Geometry check sheet. Reference: the model listing, model coordinates, mm. Face numbers are marked on the shaded views. A direction names the side the tool comes from. Coordinates: 2 decimals unless noted, no trailing zeros. Loops run counter-clockwise (first coordinate to the right, second up) from the corner with the lowest first, then second, coordinate; pieces in that order, holes last.
from build123d import *

# Parameters (mm, degrees)
BOSS_EXTRUDE1_DEPTH = 10
FILLET1_R           = 3
SKETCH2_R           = 1.4
CUT_EXTRUDE1_DEPTH  = 58.606674312


with BuildPart() as part:
    # Sketch1 → Boss-Extrude1 (new body)
    with BuildSketch(Plane(origin=(0, 0, 0), x_dir=(1, 0, 0), z_dir=(0, 1, 0))):
        with BuildLine():
            Line((7.5, -36.300826437), (7.5, -46.300826437))
            ThreePointArc((7.5, -46.300826437), (0, -53.800826437), (-7.5, -46.300826437))
            Line((-7.5, -46.300826437), (-7.5, -36.300826437))
            ThreePointArc((-7.5, -36.300826437), (-9.468913253, -22.407853181), (-15.220588235, -9.609042292))
            ThreePointArc((-15.220588235, -9.609042292), (0, 18), (15.220588235, -9.609042292))
            ThreePointArc((15.220588235, -9.609042292), (9.468913253, -22.407853181), (7.5, -36.300826437))
        make_face()
    extrude(amount=BOSS_EXTRUDE1_DEPTH)

    # Fillet1
    fillet1_edges = [part.edges().sort_by_distance(p)[0] for p in [
        (-9.468913253, 10, 22.407853181),
        (-7.5, 10, 41.300826437),
        (0, 10, 53.800826437),
        (7.5, 10, 41.300826437),
        (9.468913253, 10, 22.407853181),
        (7.5, 0, 41.300826437),
        (0, 0, 53.800826437),
        (-7.5, 0, 41.300826437),
        (-9.468913253, 0, 22.407853181),
        (0, 0, -18),
        (9.468913253, 0, 22.407853181),
        (0, 10, -18),
    ]]
    fillet(fillet1_edges, radius=FILLET1_R)

    # Sketch2 → Cut-Extrude1 (cut, through all)
    with BuildSketch(Plane(origin=(0, 10, 0), x_dir=(1, 0, 0), z_dir=(0, 1, 0))):
        with Locations(Location((0, 13.5, 0), (0, 0, 270))):
            Circle(SKETCH2_R)
        with Locations(Location((-11.691342951, -6.75, 0), (0, 0, 270))):
            Circle(SKETCH2_R)
        with Locations(Location((11.691342951, -6.75, 0), (0, 0, 270))):
            Circle(SKETCH2_R)
    extrude(amount=-CUT_EXTRUDE1_DEPTH, mode=Mode.SUBTRACT)


solid = part.part
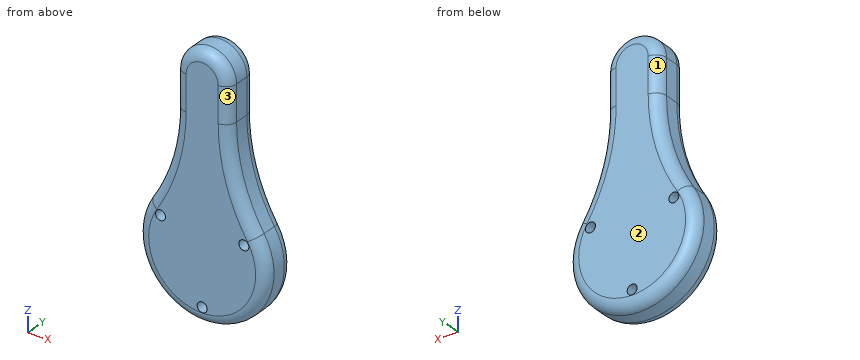
(1) Scan lines: L1, parallel to X at y = 6, z = 6.75; L2, parallel to X at y = 3.75, z = 44; L3, parallel to Z at x = -11, y = 1. Record each from-to range of solid material in increasing order.
Findings:
L1: x = -16.69 to -13.09, -10.29 to 10.29, 13.09 to 16.69
L2: x = -7.5 to 7.5
L3: z = -13.27 to 5.53, 7.97 to 15.94
(2) Gauge pin test, flat ends, axial feed: pin 1 Ø1.2 at (y, z) = (5, 42) entering from +X; pin 2 Ø6 at (x, y) = (-14.5, 7.5) entering from +Z; pin 3 Ø12 at (x, z) = (12, 35.5) entering from -Y. Record the tip position at first contact, or that the pin passes through.
Findings:
pin 1: stops at x = 7.5
pin 2: stops at z = 16.65
pin 3: stops at y = 0.4
(3) Sectioned sample at D-D on z = 6.5. State how many separate pieces and enclosed holes the cut face has, and give its area (3 significant figures).
Findings:
separate pieces: 3
enclosed holes: 0
area: 272 mm2
(4) Access from +Z, -Z, +X, -X, +Y, -Y to the whole of each face (thin tool, end or side, straight path). Record for the marked faces 1, 2 and 3.
Findings:
face 1: +Z, -X, +Y
face 2: +Z, -Z, +X, -X, +Y
face 3: +Z, +X, -Y
(5) Sectioned sample at A-A on x = 0. Record the cut outline in (y, z), and give its area (3 significant figures).
Findings:
outline: (0, -15) arc R3 ccw to (3, -18) - (7, -18) arc R3 ccw to (10, -15) - (10, -14.9) - (0, -14.9) - close; (0, -12.1) - (10, -12.1) - (10, 50.8) arc R3 ccw to (7, 53.8) - (3, 53.8) arc R3 ccw to (0, 50.8) - close
area: 682 mm2
(6) Sectioned sample at C-C on y = 4. Record the cut outline in (x, z), and give its area (3 significant figures).
Findings:
outline: (-15.22, 9.61) arc R18 ccw (long way) to (15.22, 9.61) arc R50 cw to (7.5, 36.3) - (7.5, 46.3) arc R7.5 ccw to (-7.5, 46.3) - (-7.5, 36.3) arc R50 cw to start; hole circle Ø2.8 at (-11.69, 6.75); hole circle Ø2.8 at (0, -13.5); hole circle Ø2.8 at (11.69, 6.75)
area: 1,590 mm2
(7) Sectioned sample at B-B on z = 40. Record the cut outline in (x, y), and give its area (3 significant figures).
Findings:
outline: (-7.5, 3) arc R3 ccw to (-4.5, 0) - (4.5, 0) arc R3 ccw to (7.5, 3) - (7.5, 7) arc R3 ccw to (4.5, 10) - (-4.5, 10) arc R3 ccw to (-7.5, 7) - close
area: 142 mm2
